Work out the finished part from the listing and answer in its coordinate system (mm). Round coordinates to 2 decimals unless told otherwise and drop trailing zeros. Order: outer loops, then holes, each group sorted by start corner. A loop starts at its lowest first (then second) coordinate and runs counter-clockwise, first axis right, second up. Notation, with made-up numbers: (83, 88) - (136, 88) arc R27 ccw to (136, 116) - close; hole circle Ø7 at (23.25, 17.25). An arc over 180 degrees is marked (long way). Use one line per item in the form item = value. Start each with the question number.
Q1. Find the intervals of material crossed by line 1 (Y direction, x = 43.5, z = 1.75); line 2 (X direction, y = 21.5, z = 3); line 3 (X direction, y = 19.5, z = 1.5), in increasing order. Write a range as [from, to].
Q2. The part is cut by section B-B on x = 40. Determine the outline of the cut face in (y, z).
Q3. The part is cut by section A-A on y = 10. Determine the outline of the cut face in (x, z), plus the area to 3 significant figures.
Q4. Given P1, Ø1, axis at y = 0.5, z = 3, coming from the -X side, flat-ended and moving along its own axis, determine where the tip first touches the part or whether it passes through.
from build123d import *

# Parameters (mm, degrees)
SKETCH1_W           = 102.87
SKETCH1_H           = 30.48
BOSS_EXTRUDE1_DEPTH = 1.57
FILLET1_R           = 3.935
BOSS_EXTRUDE2_DEPTH = 2
BOSS_EXTRUDE4_DEPTH = 4
BOSS_EXTRUDE5_DEPTH = 2
CHAMFER1_SIZE       = 0.4
CHAMFER1_SIZE2      = 1.492820323
CHAMFER2_SIZE       = 0.4


with BuildPart() as part:
    # Sketch1 → Boss-Extrude1 (new body)
    with BuildSketch(Plane.XY):
        with Locations((51.435, 15.24)):
            Rectangle(SKETCH1_W, SKETCH1_H)
    extrude(amount=BOSS_EXTRUDE1_DEPTH)

    # Fillet1
    fillet1_edges = [part.edges().sort_by_distance(p)[0] for p in [
        (0, 30.48, 0.785),
        (102.87, 30.48, 0.785),
        (102.87, 0, 0.785),
        (0, 0, 0.785),
    ]]
    fillet(fillet1_edges, radius=FILLET1_R)


with BuildPart() as body_2:
    # Sketch7 → Boss-Extrude2 (new body)
    with BuildSketch(Plane.XY.offset(1.57)):
        with BuildLine():
            Line((-3, 26.545), (-3, 3.935))
            ThreePointArc((-3, 3.935), (-0.968785528, -0.968785528), (3.935, -3))
            Line((3.935, -3), (98.935, -3))
            ThreePointArc((98.935, -3), (103.838785528, -0.968785528), (105.87, 3.935))
            Line((105.87, 3.935), (105.87, 26.545))
            ThreePointArc((105.87, 26.545), (103.838785528, 31.448785528), (98.935, 33.48))
            Line((98.935, 33.48), (3.935, 33.48))
            ThreePointArc((3.935, 33.48), (-0.968785528, 31.448785528), (-3, 26.545))
        make_face()
        with BuildLine():
            Line((0, 26.545), (0, 3.935))
            ThreePointArc((0, 3.935), (1.152534816, 1.152534816), (3.935, 0))
            Line((3.935, 0), (98.935, 0))
            ThreePointArc((98.935, 0), (101.717465184, 1.152534816), (102.87, 3.935))
            Line((102.87, 3.935), (102.87, 26.545))
            ThreePointArc((102.87, 26.545), (101.717465184, 29.327465184), (98.935, 30.48))
            Line((98.935, 30.48), (3.935, 30.48))
            ThreePointArc((3.935, 30.48), (1.152534816, 29.327465184), (0, 26.545))
        make_face(mode=Mode.SUBTRACT)
    extrude(amount=BOSS_EXTRUDE2_DEPTH)

    # Sketch9 → Boss-Extrude4 (add)
    with BuildSketch(Plane(origin=(0, 0, 1.57), x_dir=(-1, 0, 0), z_dir=(0, 0, -1))):
        with BuildLine():
            Line((-3.935, 33.48), (-98.935, 33.48))
            ThreePointArc((-98.935, 33.48), (-103.838785528, 31.448785528), (-105.87, 26.545))
            Line((-105.87, 26.545), (-105.87, 3.935))
            ThreePointArc((-105.87, 3.935), (-103.838785528, -0.968785528), (-98.935, -3))
            Line((-98.935, -3), (-3.935, -3))
            ThreePointArc((-3.935, -3), (0.968785528, -0.968785528), (3, 3.935))
            Line((3, 3.935), (3, 26.545))
            ThreePointArc((3, 26.545), (0.968785528, 31.448785528), (-3.935, 33.48))
        make_face()
        with BuildLine():
            Line((-98.935, 0), (-3.935, 0))
            ThreePointArc((-3.935, 0), (-1.152534816, 1.152534816), (0, 3.935))
            Line((0, 3.935), (0, 26.545))
            ThreePointArc((0, 26.545), (-1.152534816, 29.327465184), (-3.935, 30.48))
            Line((-3.935, 30.48), (-98.935, 30.48))
            ThreePointArc((-98.935, 30.48), (-101.717465184, 29.327465184), (-102.87, 26.545))
            Line((-102.87, 26.545), (-102.87, 3.935))
            ThreePointArc((-102.87, 3.935), (-101.717465184, 1.152534816), (-98.935, 0))
        make_face(mode=Mode.SUBTRACT)
    extrude(amount=BOSS_EXTRUDE4_DEPTH)

    # Sketch11 → Boss-Extrude5 (add)
    with BuildSketch(Plane.XY.offset(3.57)):
        with BuildLine():
            Line((-3, 26.545), (-3, 3.935))
            ThreePointArc((-3, 3.935), (-0.968785528, -0.968785528), (3.935, -3))
            Line((3.935, -3), (98.935, -3))
            ThreePointArc((98.935, -3), (103.838785528, -0.968785528), (105.87, 3.935))
            Line((105.87, 3.935), (105.87, 26.545))
            ThreePointArc((105.87, 26.545), (103.838785528, 31.448785528), (98.935, 33.48))
            Line((98.935, 33.48), (3.935, 33.48))
            ThreePointArc((3.935, 33.48), (-0.968785528, 31.448785528), (-3, 26.545))
        make_face()
        with BuildLine():
            Line((101.87, 3.935), (101.87, 26.545))
            ThreePointArc((101.87, 26.545), (101.010358403, 28.620358403), (98.935, 29.48))
            Line((98.935, 29.48), (3.935, 29.48))
            ThreePointArc((3.935, 29.48), (1.859641597, 28.620358403), (1, 26.545))
            Line((1, 26.545), (1, 3.935))
            ThreePointArc((1, 3.935), (1.859641597, 1.859641597), (3.935, 1))
            Line((3.935, 1), (98.935, 1))
            ThreePointArc((98.935, 1), (101.010358403, 1.859641597), (101.87, 3.935))
        make_face(mode=Mode.SUBTRACT)
    extrude(amount=-BOSS_EXTRUDE5_DEPTH)

    # Chamfer1
    chamfer1_edges = [body_2.edges().sort_by_distance(p)[0] for p in [
        (101.717465184, 1.152534816, -2.43),
        (51.435, 0, -2.43),
        (1.152534816, 1.152534816, -2.43),
        (0, 15.24, -2.43),
        (1.152534816, 29.327465184, -2.43),
        (51.435, 30.48, -2.43),
        (101.717465184, 29.327465184, -2.43),
        (102.87, 15.24, -2.43),
    ]]
    chamfer1_side = [body_2.faces().sort_by_distance(p)[0] for p in [
        (-0.156890605, 30.636890605, -2.43),
    ]]
    chamfer(chamfer1_edges, length=CHAMFER1_SIZE, length2=CHAMFER1_SIZE2, reference=chamfer1_side[0])

    # Chamfer2
    chamfer2_edges = [body_2.edges().sort_by_distance(p)[0] for p in [
        (101.010358403, 1.859641597, 3.57),
        (51.435, 1, 3.57),
        (1.859641597, 1.859641597, 3.57),
        (1, 15.24, 3.57),
        (1.859641597, 28.620358403, 3.57),
        (51.435, 29.48, 3.57),
        (101.010358403, 28.620358403, 3.57),
        (101.87, 15.24, 3.57),
        (-0.968785528, -0.968785528, 3.57),
        (51.435, -3, 3.57),
        (103.838785528, -0.968785528, 3.57),
        (105.87, 15.24, 3.57),
        (103.838785528, 31.448785528, 3.57),
        (51.435, 33.48, 3.57),
        (-0.968785528, 31.448785528, 3.57),
        (-0.968785528, 31.448785528, -2.43),
        (51.435, 33.48, -2.43),
        (103.838785528, 31.448785528, -2.43),
        (105.87, 15.24, -2.43),
        (103.838785528, -0.968785528, -2.43),
        (51.435, -3, -2.43),
        (-0.968785528, -0.968785528, -2.43),
        (-3, 15.24, -2.43),
        (-3, 15.24, 3.57),
    ]]
    chamfer(chamfer2_edges, length=CHAMFER2_SIZE)


solid = body_2.part
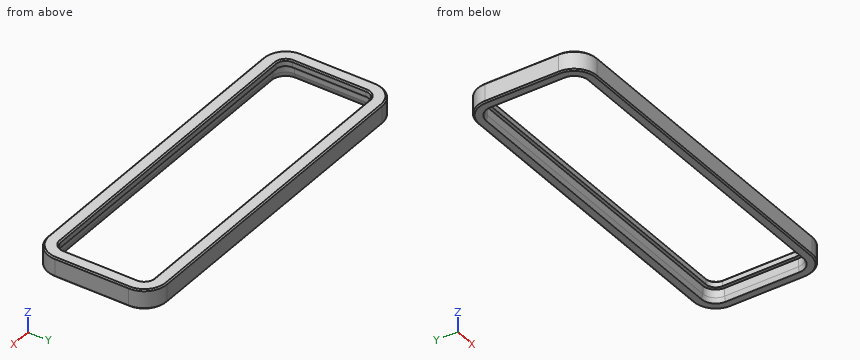
Found:
q1.line_1 = [-3, 1], [29.48, 33.48]
q1.line_2 = [-3, 1], [101.87, 105.87]
q1.line_3 = [-3, 0], [102.87, 105.87]
q2.outline = (-3, -2.03) - (-2.6, -2.43) - (-0.4, -2.43) - (0, -0.94) - (0, 1.57) - (1, 1.57) - (1, 3.17) - (0.6, 3.57) - (-2.6, 3.57) - (-3, 3.17) - close; (29.48, 1.57) - (30.48, 1.57) - (30.48, -0.94) - (30.88, -2.43) - (33.08, -2.43) - (33.48, -2.03) - (33.48, 3.17) - (33.08, 3.57) - (29.88, 3.57) - (29.48, 3.17) - close
q3.outline = (-3, -2.03) - (-2.6, -2.43) - (-0.4, -2.43) - (0, -0.94) - (0, 1.57) - (1, 1.57) - (1, 3.17) - (0.6, 3.57) - (-2.6, 3.57) - (-3, 3.17) - close; (101.87, 1.57) - (102.87, 1.57) - (102.87, -0.94) - (103.27, -2.43) - (105.47, -2.43) - (105.87, -2.03) - (105.87, 3.17) - (105.47, 3.57) - (102.27, 3.57) - (101.87, 3.17) - close
q3.area = 38.9 mm²
q4.P1 = -2.35
